Could you check a few things on this model? Use its own coordinates, in mm. Face numbers are marked on the shaded views. A direction names the side the tool comes from. Round coordinates to 2 decimals unless told otherwise and drop trailing zeros. Write each loop counter-clockwise with the first axis right and the second up, starting at its lowest first coordinate (ties: lowest second). Pieces come first, ordered by that corner, then holes. Notation, with made-up numbers: (1, 51) -> (20, 51) arc R21 ccw to (20, 80) -> close; hole circle Ø2 at (68.25, 61). An arc over 180 degrees is marked (long way). Answer in a Markdown table with one row per item.
from build123d import *

# Parameters (mm, degrees)
F0_R     = 15
F1_DEPTH = 10
F2_R     = 12.5
F3_DEPTH = 40
F4_R     = 1
F5_R     = 14.5
F6_DEPTH = 8


# Not quite as in the source:
# - a fillet or chamfer that OpenCascade refuses, or shapes differently, is made with other operations: its cross-section is extruded or revolved along the edge and cut away or added


with BuildPart() as f1:
    # F0 (on Front) → F1 (new body)
    with BuildSketch(Plane.XZ):
        with Locations((-53.2553978264, 6.2320148572)):
            Circle(F0_R)
    extrude(amount=F1_DEPTH)

    # F2 (on face) → F3 (join)
    with BuildSketch(Plane.XZ.offset(10)):
        with Locations((-53.2553978264, 6.2320148572)):
            Circle(F2_R)
    extrude(amount=F3_DEPTH)

    # F4
    f4_edges = [f1.edges().sort_by_distance(p)[0] for p in [
        (-65.755398, -50, 6.232015),
    ]]
    fillet(f4_edges, radius=F4_R)

    # F5 (on face) → F6 (join)
    with BuildSketch(Plane(origin=(0, 0, 0), x_dir=(-1, 0, 0), z_dir=(0, 1, 0))):
        with Locations((53.2553978264, 6.2320148572)):
            Circle(F5_R)
    extrude(amount=F6_DEPTH)

    # F7: fillet of radius 2 on 1 edges, made by hand

    # F7_s1 → F7_t2 (revolve, cut)
    with BuildSketch(Plane.XY.offset(6.2320148572)):
        with BuildLine():
            ThreePointArc((-38.2553978264, -1.3228756555), (-38.384569133, -0.6157688743), (-38.7553978264, 0))
            Line((-38.7553978264, 0), (-38.2553978264, 0))
            Line((-38.2553978264, 0), (-38.2553978264, -1.3228756555))
        make_face()
    revolve(axis=Axis((-53.2553978264, 0, 6.2320148572), (0, -1, 0)), mode=Mode.SUBTRACT)


solid = f1.part
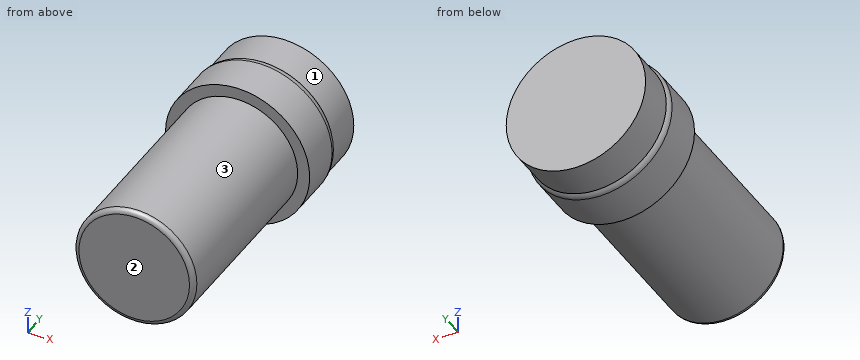
1) For pin 1 (6 mm diameter, centred on y = -28.5, z = 5, fed in from -X); pin 2 (12 mm diameter, centred on y = -9.5, z = 16, fed in from -X); pin 3 (10 mm diameter, centred on x = -63, y = -35, fed in from -Z), each with a flat end and sliding along its axis, tell me the tip position at first contact or that it passes through.
Findings:
| item | result |
|---|---|
| pin 1 | stops at x = -65.76 |
| pin 2 | stops at x = -67.77 |
| pin 3 | stops at z = -5.33 |
2) Imagine slicing it at A-A, the plane y = -2.5. Please give me the cut outline in (x, z), plus the area to 3 significant figures.
Findings:
| item | result |
|---|---|
| outline | circle Ø30 at (-53.26, 6.23) |
| area | 707 mm^2 |
3) Please list where these lines run through material, in increasing order: line 1 (Z direction, x = -53.5, y = 0); line 2 (Y direction, x = -40.75, z = 10.5); line 3 (Z direction, x = -48.25, y = -39.5).
Findings:
| item | result |
|---|---|
| line 1 | z = -8.27 to 20.73 |
| line 2 | y = -10 to 8 |
| line 3 | z = -5.22 to 17.69 |
4) For the marked faces 1, 2 and 3, which set-ups out of +Z, -Z, +X, -X, +Y, -Y let a thin tool reach every point of the face, with its end or its side?
Findings:
| item | result |
|---|---|
| face 1 | +Y |
| face 2 | +Z, -Z, +X, -X, -Y |
| face 3 | -Y |
5) Imagine slicing it at B-B, the plane y = -22. Please give me the cut outline in (x, z).
Findings:
| item | result |
|---|---|
| outline | circle Ø25 at (-53.26, 6.23) |
